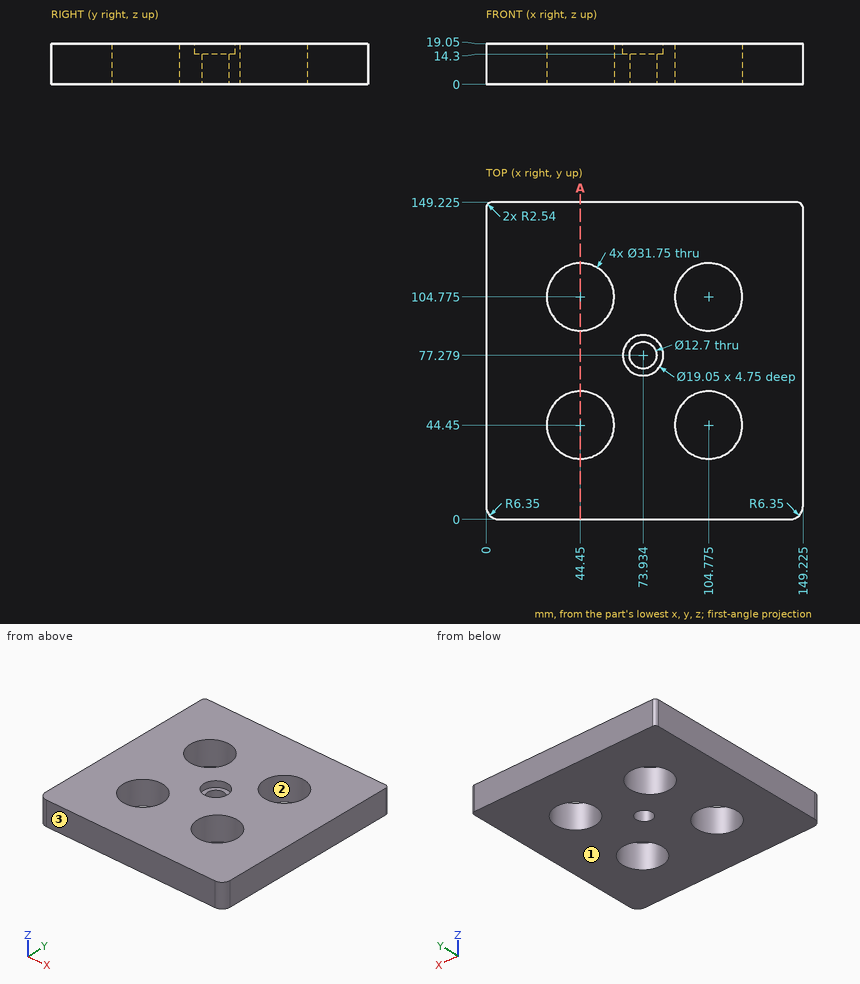
Geometry check sheet. Reference: drawing and pictorial views, mm from the part's lowest x, y, z. Give positions to 0.01 mm unless a question says otherwise; leave off trailing zeros. One line per item, written item: value. Start each with the question number.
Item 1: Material ranges on probe 1 along X at (y, z) = (105.5, 16) (1 decimal); probe 2 along X at (y, z) = (101.5, 12.25) (1 decimal); probe 3 along Y at (x, z) = (94, 9.5) (1 decimal), recorded low to high. Write a range as from..to.
Item 2: Section check A-A on x = 44.45. State how many separate pieces and enclosed holes the cut face has, then the cut area to 3 significant figures.
Item 3: Gauge pin test, flat end, axial feed: pin 1 (11.5 mm diameter, centred on x = 73.93, y = 77.28, fed in from +Z). Record the tip position at first contact, or that the pin passes through.
Item 4: Draft check along Y on the marked faces 1, 2 and 3. Enter one of: +Y half, -Y half, draft (parallel to the pull), parting line (faces both ways), or undercut.
Results list:
1. probe 1: 0..28.6, 60.3..88.9, 120.6..149.2
1. probe 2: 0..28.9, 60..89.2, 120.3..149.2
1. probe 3: 0..32.8, 56.1..93.1, 116.4..149.2
2. separate pieces: 3
2. enclosed holes: 0
2. area: 1,630 mm²
3. pin 1: through
4. face 1: draft
4. face 2: undercut
4. face 3: -Y half
